Autodesk Inventor part; units mm, degrees
ref_plane "YZ Plane" through (0, 0, 0) normal (1, 0, 0) x (0, 1, 0)
ref_plane "XZ Plane" through (0, 0, 0) normal (0, 1, 0) x (-1, 0, 0)
ref_plane "XY Plane" through (0, 0, 0) normal (0, 0, 1) x (1, 0, 0)
sketch "Sketch1" plane through (0, 6.2481, 6.7374) normal (1, 0, 0) x (0, 1, 0)
  line L0 (21.1383, 36.7567) -> (20.6141, 36.7567)
  arc A0 (24.3907, 33.5692) -> (18.0407, 33.5826) centre (21.2157, 33.5826) ccw
  arc A1 (14.8657, -15.4374) -> (16.4404, -11.3937) centre (-103.5619, 33.0092) ccw
  arc A2 (18.4214, -5.6206) -> (14.8657, -28.6257) centre (91.0657, -28.6257) ccw
  arc A3 (20.207, 36.5931) -> (4.8725, 28.8882) centre (54.3249, -50.4207) ccw
  arc A4 (18.4214, -5.6206) -> (24.3907, 33.5692) centre (-103.5619, 33.0092) ccw
  line L1 (14.8657, 1.8326) -> (14.8657, 27.2326)
  line L2 (14.8657, 1.8326) -> (14.8657, 33.5826)
  line L3 (-10.5343, 1.8326) -> (14.8657, 1.8326) construction
  line L4 (-10.5343, 1.8326) -> (-10.5343, 27.2326)
  line L5 (-10.5343, 1.8326) -> (-23.2343, 1.8326)
  line L6 (-10.5343, 1.8326) -> (-10.5395, -10.8674)
  line L7 (-10.5395, -10.8674) -> (2.1605, -10.8727)
  line L8 (21.2157, 33.5826) -> (19.8929, 33.5826)
  line L9 (14.8657, 33.5826) -> (21.2157, 33.5826)
  arc A5 (-6.7994, 20.2847) -> (-12.9991, 12.2415) centre (9.812, 1.0696) ccw
  line L10 (14.8657, 33.5826) -> (-10.5343, 33.5826)
  line L11 (2.1605, -10.8727) -> (2.1605, -17.9797)
  line L12 (2.1605, -17.9797) -> (10.4725, -17.9797)
  line L13 (2.1605, -17.9797) -> (-5.7795, -17.9797)
  line L14 (-8.9545, -14.8047) -> (-8.9545, 1.0703)
  line L15 (13.6475, -14.8047) -> (13.6475, 1.8326)
  arc A6 (-2.9466, 21.2359) -> (-8.9545, 1.0703) centre (27.8921, 1.0703) ccw
  arc A7 (4.8725, 28.8882) -> (-2.9466, 21.2359) centre (18.3119, 7.3349) ccw
  arc A8 (16.4403, 9.623) -> (23.7808, 20.5184) centre (10.0212, 21.8681) ccw
  arc A9 (18.1559, 10.6889) -> (13.6475, 1.8326) centre (24.6004, 1.8326) ccw
  arc A10 (10.4725, -17.9797) -> (13.6475, -14.8047) centre (10.4725, -14.8047) ccw
  arc A11 (-8.9545, -14.8047) -> (-5.7795, -17.9797) centre (-5.7795, -14.8047) ccw
  line L16 (2.1605, -10.8727) -> (2.1605, 1.8273)
  line L17 (13.6475, 1.8326) -> (-8.9467, 1.8326)
  point P0 (0, 0)
  point P1 (13.6475, -17.9797)
  point P2 (-8.9545, -17.9797)
  point P3 (-8.9545, -10.868)
  point P4 (19.8992, 36.4718)
  dimension "d9" = 25.4
  dimension "d7" = 12.7
  dimension "d11" = 6.35
  dimension "d12" = 6.35
  dimension "d8" = 31.75
  dimension "d10" = 25.4
  dimension "d5" = 25.4
  dimension "d6" = 12.7
  dimension "d4" = 25.4
  dimension "d3" = 19.05
  dimension "d2" = 25.4
  dimension "d1" = 3.175
  dimension "d0" = 12.7
extrude "Extrusion1" add sketch "Sketch1" along normal blind 1.5875 contours A4 A8 A9 L1 L2 L9 A0 A3 | A0 L9 L10 A3 | A9 L17 A6 A7 A3 L10 L2 L1
hole "Hole1" at (0, 21.1138, 33.9701) at (0, 8.4085, -4.1352) at (0, 8.4085, 8.5648) direction (1, 0, 0) diameter 4.7625 end through all
properties part number "sled-inner"
CAD build for the part. Positions are in the model's coordinates, mm. Coordinates: 2 decimals unless noted, no trailing zeros. Write each loop counter-clockwise with the first axis right and the second up, starting at its lowest first coordinate (ties: lowest second). Pieces come first, ordered by that corner, then holes. Notation, with made-up numbers: (1.25, 85.25) - (35.25, 85.25) arc R13 ccw to (35.25, 95.25) - close; hole circle Ø11 at (-13, 67.5). An arc over 180 degrees is marked (long way). Use a Markdown table: item, result. Add a question column.
Item 1: Band-saw the part on C-C, the plane y = 12. Give the cut face in (x, z).
Item 2: Band-saw the part on A-A, the plane x = 0.25. Give the cut face in (y, z).
Item 3: Band-saw the part on D-D, the plane y = 5.5. Give the cut face in (x, z).
Item 4: Mould opens along Y. For faces 1 (the face through (0.8, 22.56, 32.08)), 2 (the face through (0, 14, 22)), 3 (the face through (0.805, 8.461, 10.945)), 4 (the face through (0.783, 18.503, 39.777)) say: pulls with the +Y half, pulls with the -Y half, needs draft (parallel to the pull), parting line crosses it, or undercut.
Item 5: Drill centre lines: L1, parallel to Y at x = 1.2, z = 34; L2, parallel to Z at x = 0.4, y = 22.5; L3, parallel to Y at x = 1.2, z = 34.5. Where is each one in solid material? Low to high. Write a range as from..to.
Item 6: Band-saw the part on B-B, the plane y = 22. Give the cut face in (x, z).
Numbers:
| question | item | result |
|---|---|---|
| 1 | outline | (0, 8.57) - (1.59, 8.57) - (1.59, 36.17) - (0, 36.17) - close |
| 2 | outline | (-2.7, 8.57) - (6.03, 8.57) arc R2.38 cw to (10.79, 8.57) - (19.9, 8.57) arc R10.95 cw to (24.4, 17.43) arc R13.83 ccw to (30.03, 27.26) arc R127.95 ccw to (30.64, 40.31) arc R3.18 ccw to (26.46, 43.33) arc R93.47 ccw to (11.12, 35.63) arc R25.4 ccw to (3.3, 27.97) arc R36.85 ccw to start; hole circle Ø4.76 at (21.11, 33.97) |
| 3 | outline | (0, 8.57) - (1.59, 8.57) - (1.59, 30.86) - (0, 30.86) - close |
| 4 | face 1 | undercut |
| 4 | face 2 | needs draft |
| 4 | face 3 | undercut |
| 4 | face 4 | pulls with the -Y half |
| 5 | L1 | 8.81..18.73, 23.49..30.51 |
| 5 | L2 | 15.66..32.03, 35.91..41.67 |
| 5 | L3 | 9.46..18.79, 23.44..30.53 |
| 6 | outline | (0, 15.03) - (1.59, 15.03) - (1.59, 31.76) - (0, 31.76) - close; (0, 36.18) - (1.59, 36.18) - (1.59, 41.45) - (0, 41.45) - close |
